The model under review builds one solid part; all positions refer to its coordinate system, in mm. Face numbers are marked on the shaded views. A direction names the side the tool comes from. Round coordinates to 2 decimals unless told otherwise and drop trailing zeros. Order: outer loops, then holes, each group sorted by start corner. A loop starts at its lowest first (then second) coordinate and runs counter-clockwise, first axis right, second up. Notation, with made-up numbers: M 24,-22 L 66,-22 A18 ccw 66,-4 Z; hole C -1,53 d7. An arc over 180 degrees is marked long. Answer as a JSON object with one key per item and string values. Group by question number.
1. Add section D-D on x = 7. Give the number of separate pieces and of enclosed holes in the cut face, and give its area (3 significant figures).
2. Machinability: for the marked faces 4, 5, 6 and 7, which of the approach directions +Z, -Z, +X, -X, +Y, -Y give a long, thin tool a straight path to every point of the face, cutting with its end or side? Answer none if there is none.
3. To check wall thickness, follow probe 1 along X at (y, z) = (13, 5.5) (3 decimals); probe 2 along Y at (x, z) = (11.75, 5.5); probe 3 along Y at (x, z) = (-5.5, 2). State the ranges of each line that lie inside material, in increasing order. Write a range as [from, to].
4. Add section B-B on y = 2.4. State the section outline as (x, z) points (3 decimals).
5. Add section C-C on y = -4. State the section outline as (x, z) points (1 decimal), and give its area (3 significant figures).
6. Mouldability with a two-part tool opening along X and no side actions: class the marked faces 1, 2 and 3 as released by +X, released by -X, zero draft, split by the parting line, or undercut.
7. Clearance check with flat-ended pins moving along their axes: P1, Ø2, axis at x = -2.5, z = 7.5, coming from the -Y side; P2, Ø2, axis at x = 1.5, z = 6, coming from the +Y side; P3, Ø1.6, axis at x = -12, z = 5.5, coming from the +Y side. State where each tip first meets the part, or that it passes through.
8. Add section A-A on x = 0. State the section outline as (y, z) points (1 decimal), and give its area (3 significant figures).
Autodesk Inventor part; units mm, degrees
ref_plane "YZ Plane" through (0, 0, 0) normal (1, 0, 0) x (0, 1, 0)
ref_plane "XZ Plane" through (0, 0, 0) normal (0, 1, 0) x (-1, 0, 0)
ref_plane "XY Plane" through (0, 0, 0) normal (0, 0, 1) x (1, 0, 0)
sketch "Sketch1" plane through (0, 0, 0) normal (0, 0, 1) x (1, 0, 0)
  line L0 (-13.425, -7.5) -> (13.425, -7.5)
  line L1 (13.425, -7.5) -> (13.425, 7.5)
  line L2 (13.425, 7.5) -> (-13.425, 7.5)
  line L3 (-13.425, 7.5) -> (-13.425, -7.5)
  line L4 (-13.425, -7.5) -> (13.425, 7.5) construction
  line L5 (13.425, -7.5) -> (-13.425, 7.5) construction
  point P0 (0, 0)
  dimension "d0" = 26.85
  dimension "d1" = 15
extrude "Extrusion1" add sketch "Sketch1" along normal blind 8.91
sketch "Sketch2" plane through (0, 0, 8.91) normal (0, 0, 1) x (1, 0, 0)
  line L0 (-13.425, -7.5) -> (13.425, -7.5)
  line L1 (-6.315, -7.5) -> (6.315, -7.5)
  line L2 (6.315, -7.5) -> (6.315, -4.5)
  line L3 (6.315, -4.5) -> (-6.315, -4.5)
  line L4 (-6.315, -4.5) -> (-6.315, -7.5)
  line L5 (-13.425, 7.5) -> (-13.425, -7.5)
  line L6 (13.425, -7.5) -> (13.425, 7.5)
  point P0 (0, 0)
  dimension "d4" = 7.11
  dimension "d5" = 7.11
  dimension "d6" = 3
extrude "Extrusion2" cut sketch "Sketch2" against normal through all
fillet "Fillet1" radius 1 6 edges at (-6.315, -4.5, 4.455) (6.315, -4.5, 4.455) (6.315, -7.5, 4.455) (-6.315, -7.5, 4.455) (-13.425, -7.5, 4.455) (13.425, -7.5, 4.455)
hole "Hole1" at (-9.87, -7.5, 4.455) direction (0, 1, 0) diameter 2.459 depth 5.05 tip angle 118
hole "Hole2" at (9.87, -7.5, 4.455) direction (0, 1, 0) diameter 2.459 depth 5.05 tip angle 118
sketch "Sketch3" plane through (-13.425, 7.5, 0) normal (-1, 0, 0) x (0, 0, 1)
  circle A0 centre (4.455, -5.1) radius 3.1
  line L0 (6.8136, -2) -> (2.7173, -2)
  line L1 (0, -15) -> (8.91, -15)
  point P0 (0, -7.5)
  point P1 (4.455, -15)
  dimension "d28" = 6.2
  dimension "d29" = 13
extrude "Extrusion3" cut sketch "Sketch3" against normal through all
sketch "Sketch4" plane through (-13.425, 7.5, 0) normal (-1, 0, 0) x (0, 0, 1)
  circle A0 centre (1.2775, -9.6) radius 1
  line L0 (0, -15) -> (8.91, -15)
  point P0 (0, -7.5)
  dimension "d32" = 2
  dimension "d33" = 5.4
extrude "Extrusion4" cut sketch "Sketch4" against normal through all
sketch "Sketch5" plane through (0, 0, 8.91) normal (0, 0, 1) x (1, 0, 0)
  line L0 (13.425, 7.5) -> (-13.425, 7.5)
  line L1 (-5.315, -4.5) -> (5.315, -4.5)
  line L2 (-7, 11.5) -> (-7, 7.5)
  line L3 (13.425, -6.5) -> (13.425, 7.5)
  line L4 (13.425, 14.5) -> (6.3246, 14.5)
  line L5 (7, 11.5) -> (13.425, 11.5) construction
  line L6 (7.315, -7.5) -> (12.425, -7.5)
  line L7 (13.425, 7.5) -> (13.425, 10.87)
  line L8 (13.425, 12.13) -> (13.425, 14.5)
  arc A0 (6.3246, 14.5) -> (-7, 11.5) centre (0, 11.5) ccw
  line L9 (-7, 7.5) -> (13.425, 7.5)
  line L10 (13.425, 12.13) -> (13.425, 10.87)
  point P0 (0, 0)
  dimension "d40" = 22
extrude "Extrusion5" add sketch "Sketch5" against normal up to surface (8.91 mm away)
sketch "Sketch6" plane through (0, 0, 8.91) normal (0, 0, 1) x (1, 0, 0)
  arc A0 (6.3246, 14.5) -> (-7, 11.5) centre (0, 11.5) ccw
  circle A1 centre (0, 11.5) radius 4
  point P0 (0, 0)
  dimension "d43" = 8
extrude "Extrusion6" cut sketch "Sketch6" against normal through all
sketch "Sketch7" plane through (0, 0, 8.91) normal (0, 0, 1) x (1, 0, 0)
  line L0 (2.5936, 12.15) -> (18.1554, 12.15)
  line L1 (18.1554, 12.15) -> (18.1554, 10.85)
  line L2 (18.1554, 10.85) -> (2.5936, 10.85)
  line L3 (2.5936, 10.85) -> (2.5936, 12.15)
  circle A0 centre (0, 11.5) radius 4 construction
  point P0 (0, 0)
  point P1 (2.5936, 11.5)
  dimension "d46" = 1.3
extrude "Extrusion7" cut sketch "Sketch7" against normal through all
fillet "Fillet2" radius 1 1 edges at (-7, 7.5, 4.455)
hole "Hole3" at (9.8748, 14.5, 4.455) direction (0, -1, 0) diameter 3 depth 5.8 tip angle 118
thread "Thread1"
hole "Hole4" at (0, -4.5, 4.455) direction (0, 1, 0) diameter 2.013 depth 6.35 tip angle 118
equation "\"d5\" = d4"
properties part number "hotend" material "Aluminum"
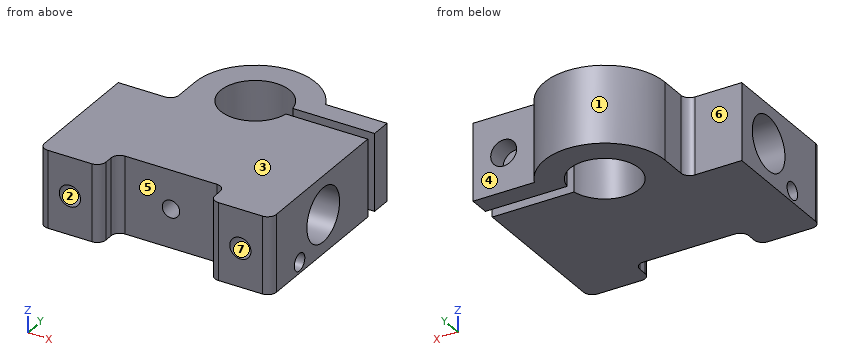
Recorded:
{
 "1": {"separate pieces": "2", "enclosed holes": "2", "area": "151 mm²"},
 "2": {"face 4": "+Z, -Z, +X, +Y", "face 5": "+Z, -Z, -Y", "face 6": "+Z, -Z, -X, +Y", "face 7": "-Y"},
 "3": {"probe 1": "x = [-6.837, -3.708], [3.708, 8.799], [10.951, 13.425]", "probe 2": "y = [-7.5, -0.52], [5.32, 10.85], [12.15, 14.5]", "probe 3": "y = [-4.52, -2.79], [-1.41, 0.51], [4.29, 15.83]"},
 "4": {"outline": "M -13.425,0 L 13.425,0 L 13.425,1.355 L -13.425,1.355 Z; M -13.425,7.555 L 13.425,7.555 L 13.425,8.91 L -13.425,8.91 Z"},
 "5": {"outline": "M -13.4,0 L 13.4,0 L 13.4,8.9 L -13.4,8.9 Z; hole C -9.9,4.5 d2.5; hole C 0,4.5 d2; hole C 9.9,4.5 d2.5", "area": "227 mm²"},
 "6": {"face 1": "split by the parting line", "face 2": "undercut", "face 3": "zero draft"},
 "7": {"P1": "stops at y = -4.5", "P2": "stops at y = 18.48", "P3": "stops at y = 7.5"},
 "8": {"outline": "M -4.5,0 L 7.5,0 L 7.5,8.9 L -4.5,8.9 L -4.5,5.5 L -0.5,5.5 A3.1 cw long -0.5,3.4 L -4.5,3.4 Z; M 15.5,0 L 18.5,0 L 18.5,8.9 L 15.5,8.9 Z; hole C -2.1,1.3 d2", "area": "92.6 mm²"}
}
